Check sheet for the drawn part. Datum: minimum x, y, z corner. Units: mm. A direction names the side the tool comes from. Give positions to 0.01 mm unless a question says otherwise; leave off trailing zeros. Write each loop counter-clockwise with the first axis right and the second up, starting at its lowest first coordinate (ties: lowest second). Pieces come first, ordered by that corner, then holes. Notation, with made-up numbers: (59, 39.5) - (71, 39.5) arc R19 ccw to (71, 75.5) - close; hole circle Ø2 at (-19.5, -32). An arc over 180 degrees is marked (long way). Answer as a JSON object with one key per item and string values. Group by question number.
Item 1: Sectioned sample at C-C, the plane x = 15.5. Record the boundary of the cut face in (y, z).
Item 2: Draft check along X on the marked faces 1, 2 and 3. Enter one of: +X half, -X half, draft (parallel to the pull), parting line (faces both ways), or undercut.
Item 3: Scan lines: line 1 along Y through (x, z) = (40.75, 20); line 2 along Y through (x, z) = (20, 39.5); line 3 along Z through (x, y) = (37, 140). Record each from-to range of solid material in increasing order. Write a range as [from, to].
Item 4: Tool access check on the marked faces 4, 5 and 6. Record the directions out of +Z, -Z, +X, -X, +Y, -Y that give a thin tool (end or side, any length) a straight path to the whole face; none if there is none.
Item 5: Sectioned sample at A-A, the plane z = 31.5. Record the boundary of the cut face in (x, y).
Item 6: Go/stop test with flat-tipped pins: pin 1 (2 mm diameter, centred on x = 7, z = 72, fed in from -Y); pin 2 (16 mm diameter, centred on x = 9, z = 51.5, fed in from +Y); pin 3 (12 mm diameter, centred on x = 20, y = 20, fed in from +Z); pin 4 (12 mm diameter, centred on x = 5, y = 18, fed in from +Z). Record where each tip stops, or that it passes through.
Item 7: Sectioned sample at D-D, the plane x = 7.5. Record the boundary of the cut face in (y, z), and give its area (3 significant figures).
Item 8: Sectioned sample at B-B, the plane y = 80. Record the boundary of the cut face in (x, z), and give its area (3 significant figures).
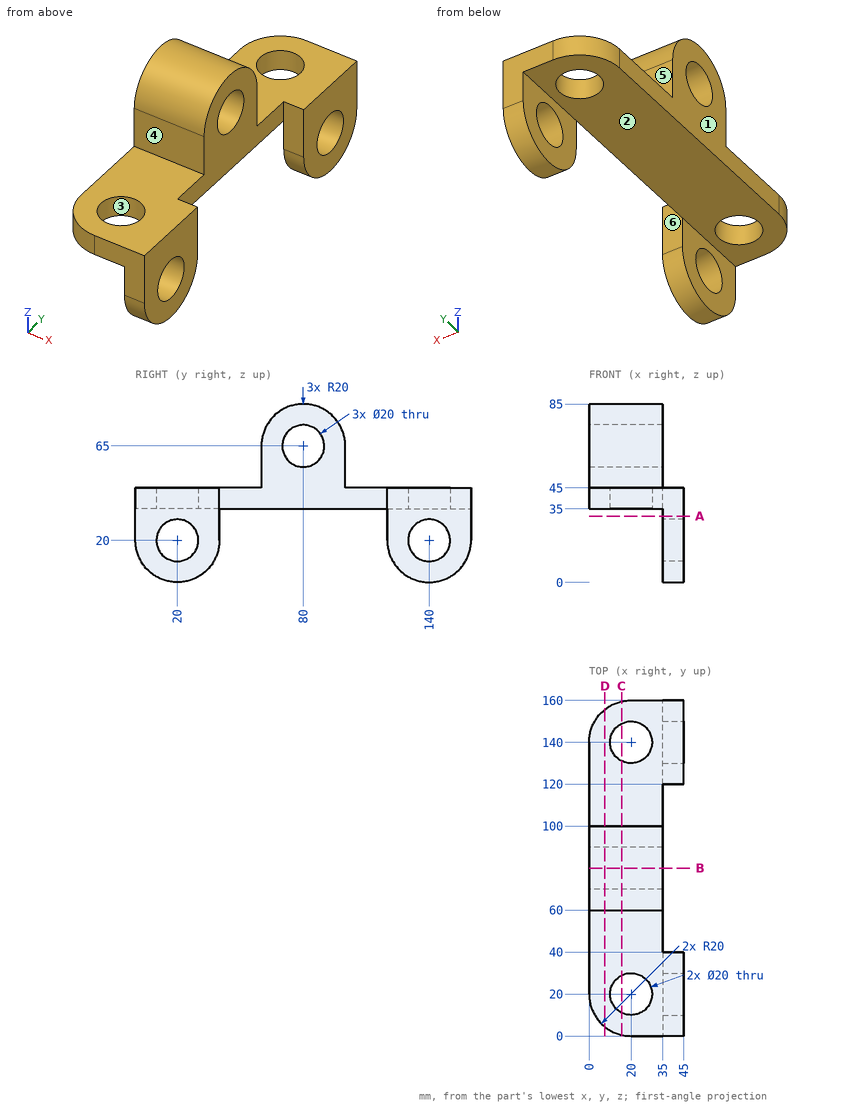
Geometry check:
{
 "1": {"outline": "(0.51, 35) - (11.07, 35) - (11.07, 45) - (0.51, 45) - close; (28.93, 35) - (131.07, 35) - (131.07, 45) - (100, 45) - (100, 65) arc R20 ccw to (60, 65) - (60, 45) - (28.93, 45) - close; (148.93, 35) - (159.49, 35) - (159.49, 45) - (148.93, 45) - close; hole circle Ø20 at (80, 65)"},
 "2": {"face 1": "-X half", "face 2": "draft", "face 3": "undercut"},
 "3": {"line 1": "[0, 10], [30, 40], [120, 130], [150, 160]", "line 2": "[0, 10], [30, 130], [150, 160]", "line 3": "[0, 10], [30, 45]"},
 "4": {"face 4": "+Z, +X, -X, -Y", "face 5": "+Z, +X, -X, +Y", "face 6": "+Z, -Z, +X"},
 "5": {"outline": "(35, 0) - (45, 0) - (45, 40) - (35, 40) - close; (35, 120) - (45, 120) - (45, 160) - (35, 160) - close"},
 "6": {"pin 1": "y = 60.92", "pin 2": "y = 158.97", "pin 3": "through", "pin 4": "z = 45"},
 "7": {"outline": "(4.39, 35) - (155.61, 35) - (155.61, 45) - (100, 45) - (100, 65) arc R20 ccw to (60, 65) - (60, 45) - (4.39, 45) - close; hole circle Ø20 at (80, 65)", "area": "2,630 mm^2"},
 "8": {"outline": "(0, 35) - (35, 35) - (35, 55) - (0, 55) - close; (0, 75) - (35, 75) - (35, 85) - (0, 85) - close", "area": "1,050 mm^2"}
}
